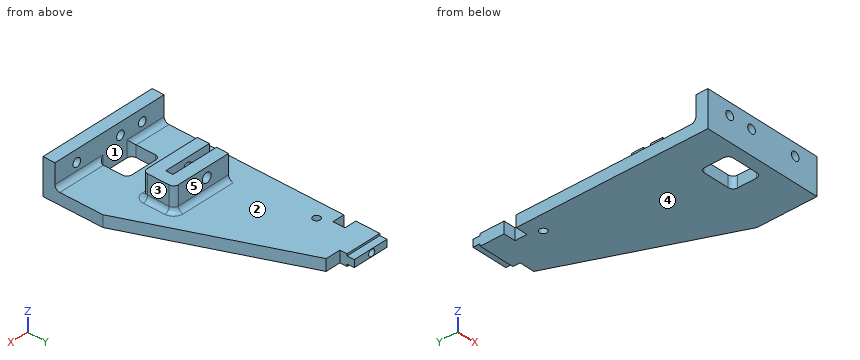
from build123d import *

# Parameters (mm, degrees)
SKETCH_1_R          = 1.5
EXTRUDE_1_DEPTH     = 4.8
SKETCH_2_W          = 50
SKETCH_2_H          = 15
SKETCH_2_R          = 1.75
EXTRUDE_2_DEPTH     = 5
EXTRUDE_3_DEPTH     = 10
SKETCH_5_R          = 2
CUT_EXTRUDE_1_DEPTH = 20
FILLET_1_R          = 2
FILLET_2_R          = 2
FILLET_3_R          = 2
SKETCH_6_W          = 15
SKETCH_6_H          = 3
EXTRUDE_5_DEPTH     = 3
SKETCH_7_R          = 1.4
CUT_EXTRUDE_2_DEPTH = 5
CUT_EXTRUDE_3_DEPTH = 73.079801494


with BuildPart() as part:
    # 草图1 → 凸台-拉伸1 (new body)
    with BuildSketch(Plane.XY):
        Polygon((-23.337979748, 53.186059405), (-23.337979748, 63.186059405), (-3.337979748, 63.186059405), (26.662020252, -6.813940595), (26.662020252, -26.813940595), (6.662020252, -26.813940595), (6.662020252, -14.813940595), (-8.337979748, -14.813940595), (-8.337979748, -26.813940595), (-23.337979748, -26.813940595), (-23.337979748, -6.813940595), (-23.337979748, 48.186059405), (-18.337979748, 48.186059405), (-18.337979748, 53.186059405), align=None)
        with Locations((-16.337979748, 43.186059405)):
            Circle(SKETCH_1_R, mode=Mode.SUBTRACT)
    extrude(amount=EXTRUDE_1_DEPTH)

    # 草图2 → 凸台-拉伸2 (add)
    with BuildSketch(Plane.XZ.offset(26.813940595)):
        with Locations((1.662020252, 7.5)):
            Rectangle(SKETCH_2_W, SKETCH_2_H)
        with Locations(Location((-13.337979748, 10, 0), (0, 0, 270))):
            Circle(SKETCH_2_R, mode=Mode.SUBTRACT)
        with Locations(Location((16.662020252, 10, 0), (0, 0, 270))):
            Circle(SKETCH_2_R, mode=Mode.SUBTRACT)
        with Locations(Location((-3.337979748, 10, 0), (0, 0, 270))):
            Circle(SKETCH_2_R, mode=Mode.SUBTRACT)
    extrude(amount=EXTRUDE_2_DEPTH)

    # 草图4 → 凸台-拉伸3 (add)
    with BuildSketch(Plane.XY.offset(4.8)):
        Polygon((11.662020252, 9.186059405), (11.662020252, -3.813940595), (-13.337979748, -3.813940595), (-13.337979748, 1.186059405), (6.662020252, 1.186059405), (6.662020252, 4.186059405), (-3.337979748, 4.186059405), (-13.337979748, 4.186059405), (-13.337979748, 9.186059405), align=None)
    extrude(amount=EXTRUDE_3_DEPTH)

    # 草图5 → 切除-拉伸1 (cut)
    with BuildSketch(Plane(origin=(0, 9.186059405, 0), x_dir=(1, 0, 0), z_dir=(0, 1, 0))):
        with Locations(Location((-3.337979748, -10.8, 0), (0, 0, 270))):
            Circle(SKETCH_5_R)
    extrude(amount=-CUT_EXTRUDE_1_DEPTH, mode=Mode.SUBTRACT)

    # 圆角1
    fillet_1_edges = [part.edges().sort_by_distance(p)[0] for p in [
        (11.662020252, -3.813940595, 9.8),
        (11.662020252, 9.186059405, 9.8),
    ]]
    fillet(fillet_1_edges, radius=FILLET_1_R)

    # 圆角2
    fillet_2_edges = [part.edges().sort_by_distance(p)[0] for p in [
        (-1.837979748, 9.186059405, 4.8),
        (11.076233814, -3.228154158, 4.8),
        (11.076233814, 8.600272967, 4.8),
        (-1.837979748, -3.813940595, 4.8),
        (11.662020252, 2.686059405, 4.8),
    ]]
    fillet(fillet_2_edges, radius=FILLET_2_R)

    # 圆角3
    fillet_3_edges = [part.edges().sort_by_distance(p)[0] for p in [
        (-15.837979748, -26.813940595, 4.8),
        (6.662020252, -26.813940595, 2.4),
        (6.662020252, -14.813940595, 2.4),
        (-8.337979748, -14.813940595, 2.4),
        (-8.337979748, -26.813940595, 2.4),
        (16.662020252, -26.813940595, 4.8),
    ]]
    fillet(fillet_3_edges, radius=FILLET_3_R)

    # 草图6 → 凸台-拉伸5 (add)
    with BuildSketch(Plane(origin=(0, 63.186059405, 0), x_dir=(1, 0, 0), z_dir=(0, 1, 0))):
        with Locations((-15.837979748, -2.5)):
            Rectangle(SKETCH_6_W, SKETCH_6_H)
    extrude(amount=EXTRUDE_5_DEPTH)

    # 草图7 → 切除-拉伸2 (cut)
    with BuildSketch(Plane(origin=(0, 66.186059405, 0), x_dir=(1, 0, 0), z_dir=(0, 1, 0))):
        with Locations(Location((-16.337979748, -2.5, 0), (0, 0, 270))):
            Circle(SKETCH_7_R)
    extrude(amount=-CUT_EXTRUDE_2_DEPTH, mode=Mode.SUBTRACT)

    # 草图8 → 切除-拉伸3 (cut, through all)
    with BuildSketch(Plane.XY.offset(4.8)):
        Polygon((-8.337979748, 63.186059405), (-8.337979748, 60.186059405), (-2.052265462, 60.186059405), (-3.337979748, 63.186059405), align=None)
    extrude(amount=-CUT_EXTRUDE_3_DEPTH, mode=Mode.SUBTRACT)


solid = part.part
Read the model definition and answer for the solid it produces. Units are mm, in the model's axes. Face numbers are marked on the shaded views. A direction names the side the tool comes from. Round coordinates to 2 decimals unless told otherwise and drop trailing zeros. Write each loop counter-clockwise with the first axis right and the second up, starting at its lowest first coordinate (ties: lowest second). Pieces come first, ordered by that corner, then holes. Notation, with made-up numbers: (15.25, 5) - (55.25, 5) arc R22 cw to (55.25, 15) - close; hole circle Ø4 at (58.5, 86). An arc over 180 degrees is marked (long way). One line per question, with ' | ' between items. Start each with the question number.
1. Section A-A (x = 3.5) is taken. Determine the outline of the cut face in (y, z).
2. Section C-C (y = 6) is taken. Determine the outline of the cut face in (x, z).
3. Each of these flat-tipped pins is pushed along its axis until it touches: pin 1 (2 mm diameter, centred on x = -4.5, z = 3.5, fed in from +Y); pin 2 (5 mm diameter, centred on y = 47, z = 7.5, fed in from -X); pin 3 (5.5 mm diameter, centred on y = 62, z = 3, fed in from +X); pin 4 (5.5 mm diameter, centred on y = 7, z = 12, fed in from -X). Where does it stop, or does it pass through?
4. Find the intervals of material crossed by probe 1 along X at (y, z) = (-29.5, 10); probe 2 along Y at (x, z) = (0, 10.75); probe 3 along X at (y, z) = (6.5, 10.8), in increasing order. Write a range as [from, to].
5. For the marked faces 4 and 5, determine the directions among +Z, -Z, +X, -X, +Y, -Y from which every point of the face is accessible in a straight line to the end or side of a thin tool.
6. For a pull along X with two mould halves and no side action, classify the marked faces 1, 2 and 3 as +X half, -X half, draft (parallel to the pull), parting line (faces both ways), or undercut.
7. Section D-D (x = 21.5) is taken. Determine the outline of the cut face in (y, z), and give its area (3 significant figures).
8. Section B-B (z = 10.8) is taken. Give the number of separate pieces and of enclosed holes in the cut face, and give its area (3 significant figures).
Filled in:
1) outline: (-31.81, 0) - (-26.81, 0) - (-26.81, 15) - (-31.81, 15) - close; (-14.81, 0) - (47.23, 0) - (47.23, 4.8) - (11.19, 4.8) arc R2 cw to (9.19, 6.8) - (9.19, 14.8) - (4.19, 14.8) - (4.19, 4.8) - (1.19, 4.8) - (1.19, 14.8) - (-3.81, 14.8) - (-3.81, 6.8) arc R2 cw to (-5.81, 4.8) - (-14.81, 4.8) - close
2) outline: (-23.34, 0) - (21.17, 0) - (21.17, 4.8) - (13.66, 4.8) arc R2 cw to (11.66, 6.8) - (11.66, 14.8) - (-13.34, 14.8) - (-13.34, 4.8) - (-23.34, 4.8) - close; hole circle Ø4 at (-3.34, 10.8)
3) pin 1: y = 60.19 | pin 2: through | pin 3: x = -1.65 | pin 4: x = -13.34
4) probe 1: [-23.34, -15.09], [-11.59, -5.09], [-1.59, 14.91], [18.41, 26.66] | probe 2: [-31.81, -26.81], [-3.81, 1.19], [4.19, 9.19] | probe 3: [-13.34, -5.34], [-1.34, 11.66]
5) face 4: -Z, +X, -X, +Y, -Y | face 5: +Z, +X, -X, +Y
6) face 1: undercut | face 2: draft | face 3: +X half
7) outline: (-31.81, 0) - (5.23, 0) - (5.23, 4.8) - (-24.81, 4.8) arc R2 cw to (-26.81, 6.8) - (-26.81, 15) - (-31.81, 15) - close | area: 230 mm²
8) separate pieces: 7 | enclosed holes: 0 | area: 427 mm²
